Could you check a few things on this model? Use its own coordinates, in mm. Face numbers are marked on the shaded views. A direction names the side the tool comes from. Coordinates: 2 decimals unless noted, no trailing zeros. Loops run counter-clockwise (first coordinate to the right, second up) from the corner with the lowest first, then second, coordinate; pieces in that order, holes last.
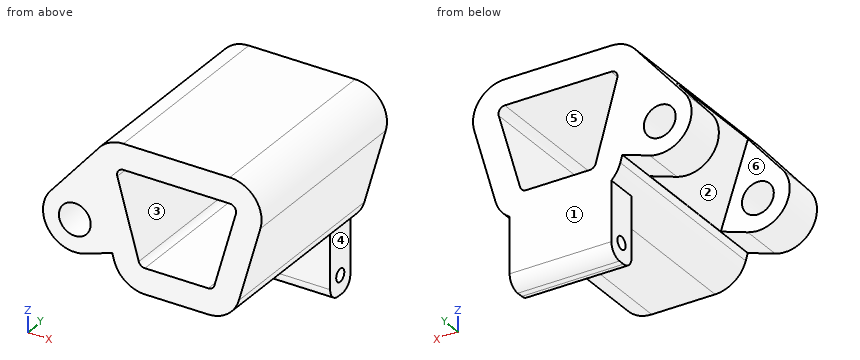
from build123d import *

# Parameters (mm, degrees)
BOSS_EXTRUDE1_DEPTH             = 31
SKETCH2_W                       = 16
SKETCH2_H                       = 5
BOSS_EXTRUDE2_DEPTH             = 10
BOSS_EXTRUDE2_DIRECTION_2_REACH = 42.293
SKETCH3_R                       = 1
CUT_EXTRUDE1_DEPTH              = 44.306250579
FILLET1_R                       = 2
SKETCH4_R                       = 2.5
BOSS_EXTRUDE3_DEPTH             = 31
SKETCH6_W                       = 18.969126519
SKETCH6_H                       = 17.5
CUT_EXTRUDE2_DEPTH              = 43.163504997


with BuildPart() as part:
    # Sketch1 → Boss-Extrude1 (new body)
    with BuildSketch(Plane(origin=(0, 0, 0), x_dir=(1, 0, 0), z_dir=(0, 1, 0))):
        with BuildLine():
            Line((-8.359903733, -11), (8.359903733, -11))
            ThreePointArc((8.359903733, -11), (12.345417465, -9.01921849), (13.173158433, -4.646272115))
            Line((13.173158433, -4.646272115), (9.798158433, 7.353727885))
            ThreePointArc((9.798158433, 7.353727885), (8.004122222, 9.985513732), (4.984903733, 11))
            Line((4.984903733, 11), (-4.984903733, 11))
            ThreePointArc((-4.984903733, 11), (-8.004122222, 9.985513732), (-9.798158433, 7.353727885))
            Line((-9.798158433, 7.353727885), (-13.173158433, -4.646272115))
            ThreePointArc((-13.173158433, -4.646272115), (-12.345417465, -9.01921849), (-8.359903733, -11))
        make_face()
        with BuildLine():
            Line((5.947554673, 6.270745577), (9.322554673, -5.729254423))
            ThreePointArc((9.322554673, -5.729254423), (9.157006479, -6.603843698), (8.359903733, -7))
            Line((8.359903733, -7), (-8.359903733, -7))
            ThreePointArc((-8.359903733, -7), (-9.157006479, -6.603843698), (-9.322554673, -5.729254423))
            Line((-9.322554673, -5.729254423), (-5.947554673, 6.270745577))
            ThreePointArc((-5.947554673, 6.270745577), (-5.588747431, 6.797102746), (-4.984903733, 7))
            Line((-4.984903733, 7), (4.984903733, 7))
            ThreePointArc((4.984903733, 7), (5.588747431, 6.797102746), (5.947554673, 6.270745577))
        make_face(mode=Mode.SUBTRACT)
    extrude(amount=BOSS_EXTRUDE1_DEPTH)

    # Sketch2 → Boss-Extrude2 (add)
    with BuildSketch(Plane(origin=(0, 0, -11), x_dir=(-1, 0, 0), z_dir=(0, 0, -1))):
        with Locations((0.398573677, 28.5)):
            Rectangle(SKETCH2_W, SKETCH2_H)
    extrude(amount=BOSS_EXTRUDE2_DEPTH)

    # Boss-Extrude2 direction 2: up to this face of the body (flat: up to its plane)
    boss_extrude2_direction_2_end = Plane(part.part.faces().sort_by_distance((0, 15.5, -7))[0])
    # Sketch2 → Boss-Extrude2 direction 2 (add, up to the picked face)
    with BuildSketch(Plane(origin=(0, 0, -11), x_dir=(-1, 0, 0), z_dir=(0, 0, -1)), mode=Mode.PRIVATE) as boss_extrude2_direction_2_sk1:
        with Locations((0.398573677, 28.5)):
            Rectangle(SKETCH2_W, SKETCH2_H)
    boss_extrude2_direction_2_tool1 = split(extrude(boss_extrude2_direction_2_sk1.sketch, amount=-BOSS_EXTRUDE2_DIRECTION_2_REACH, mode=Mode.PRIVATE), bisect_by=boss_extrude2_direction_2_end, keep=Keep.BOTH, mode=Mode.PRIVATE)
    add(boss_extrude2_direction_2_tool1.solids().sort_by(Axis((-0.398574, 28.5, -11), (0, 0, 1)))[0])

    # Sketch3 → Cut-Extrude1 (cut, through all)
    with BuildSketch(Plane.ZY.offset(8.398573677)):
        with Locations((-18, 28.5)):
            Circle(SKETCH3_R)
    extrude(amount=-CUT_EXTRUDE1_DEPTH, mode=Mode.SUBTRACT)

    # Fillet1
    fillet1_edges = [part.edges().sort_by_distance(p)[0] for p in [
        (-0.398573677, 31, -21),
        (-0.398573677, 26, -21),
    ]]
    fillet(fillet1_edges, radius=FILLET1_R)

    # Sketch4 → Boss-Extrude3 (add, through all)
    with BuildSketch(Plane(origin=(0, 31, 0), x_dir=(1, 0, 0), z_dir=(0, 1, 0))):
        with BuildLine():
            Line((-19.535533906, -0.596593374), (-12.345417465, -9.01921849))
            Line((-12.345417465, -9.01921849), (-10.109189958, 6.247838019))
            Line((-10.109189958, 6.247838019), (-14.420879995, 7.683029487))
            ThreePointArc((-14.420879995, 7.683029487), (-20.253813291, 5.566690993), (-19.535533906, -0.596593374))
        make_face()
        with Locations(Location((-16, 2.938940532, 0), (0, 0, 270))):
            Circle(SKETCH4_R, mode=Mode.SUBTRACT)
    extrude(amount=-BOSS_EXTRUDE3_DEPTH)

    # Sketch6 → Cut-Extrude2 (cut, through all)
    with BuildSketch(Plane(origin=(0.863884459, 0, -2.595334559), x_dir=(-0.9488177909602633, 0, -0.31582400092026913), z_dir=(0.31582400092026913, 0, -0.9488177909602633))):
        with Locations((21.109272612, 15.5)):
            Rectangle(SKETCH6_W, SKETCH6_H)
    extrude(amount=-CUT_EXTRUDE2_DEPTH, mode=Mode.SUBTRACT)


solid = part.part
(1) Imagine slicing it at B-B, the plane z = -18. Write out the boundary of the cut face in (x, y), and give its area (3 significant figures).
Answers:
outline: (-8.4, 26) - (7.6, 26) - (7.6, 27.5) - (-8.4, 27.5) - close; (-8.4, 29.5) - (7.6, 29.5) - (7.6, 31) - (-8.4, 31) - close
area: 48.0 mm2
(2) Imagine slicing it at D-D, the plane y = 21. Write out the boundary of the cut face in (x, z), and give its area (3 significant figures).
Answers:
outline: (-14.44, 6.57) - (-10.17, -6.27) - (-10.11, -6.25) - (-9.8, -7.35) arc R5 ccw to (-4.98, -11) - (4.98, -11) arc R5 ccw to (9.8, -7.35) - (13.17, 4.65) arc R5 ccw to (8.36, 11) - (-8.36, 11) arc R5 ccw to (-12.35, 9.02) - close; hole (-9.32, 5.73) - (-5.95, -6.27) arc R1 ccw to (-4.98, -7) - (4.98, -7) arc R1 ccw to (5.95, -6.27) - (9.32, 5.73) arc R1 ccw to (8.36, 7) - (-8.36, 7) arc R1 ccw to start
area: 288 mm2
(3) For pin 1 (2 mm diameter, centred on y = 19.5, z = 0, fed in from -X); pin 2 (4 mm diameter, centred on y = 28.5, z = -12.5, fed in from -X); pin 3 (6 mm diameter, centred on x = -14.5, y = 6, fed in from -Z), each with a flat end and sliding along its axis, tell me the tip position at first contact or that it passes through.
Answers:
pin 1: stops at x = -12.58
pin 2: stops at x = -8.4
pin 3: stops at z = -7.94
(4) Imagine slicing it at A-A, the plane x = 2. Write out the boundary of the cut face in (y, z).
Answers:
outline: (0, -11) - (26, -11) - (26, -19) arc R2 ccw to (28, -21) - (29, -21) arc R2 ccw to (31, -19) - (31, -7) - (0, -7) - close; (0, 7) - (31, 7) - (31, 11) - (0, 11) - close; hole circle Ø2 at (28.5, -18)
(5) Which directions (+Z, -Z, +X, -X, +Y, -Y) give clear straight access to the entire face, cutting with the end or side of a thin tool? Please do the marked faces 4, 5 and 6.
Answers:
face 4: -Z, +X, +Y, -Y
face 5: +Y, -Y
face 6: -Z, -X
(6) I need wall thicknesses on probe 1 along Z at (x, y) = (-1, 17); probe 2 along Y at (x, z) = (-1, -18); probe 3 along Y at (x, z) = (-6.5, -12). Which ranges of each line are inside material? Lowest first, please.
Answers:
probe 1: z = -11 to -7, 7 to 11
probe 2: y = 26 to 27.5, 29.5 to 31
probe 3: y = 26 to 31
(7) We'd pull the mould along X, two halves only. Please class the marked faces 1, 2 and 3: +X half, -X half, draft (parallel to the pull), parting line (faces both ways), or undercut.
Answers:
face 1: draft
face 2: -X half
face 3: undercut
(8) Imagine slicing it at C-C, the plane y = 28.5. Write out the boundary of the cut face in (x, z).
Answers:
outline: (-19.54, 0.6) arc R5 ccw to (-14.42, -7.68) - (-10.11, -6.25) - (-9.8, -7.35) arc R5 ccw to (-8.4, -9.65) - (-8.4, -17) - (7.6, -17) - (7.6, -10.26) arc R5 ccw to (9.8, -7.35) - (13.17, 4.65) arc R5 ccw to (8.36, 11) - (-8.36, 11) arc R5 ccw to (-12.35, 9.02) - close; (-8.4, -21) - (7.6, -21) - (7.6, -19) - (-8.4, -19) - close; hole circle Ø5 at (-16, -2.94); hole (-9.32, 5.73) - (-5.95, -6.27) arc R1 ccw to (-4.98, -7) - (4.98, -7) arc R1 ccw to (5.95, -6.27) - (9.32, 5.73) arc R1 ccw to (8.36, 7) - (-8.36, 7) arc R1 ccw to start
